```python
from build123d import *

# Parameters (mm, degrees)
SKETCH2_W           = 16
SKETCH2_H           = 14
BOSS_EXTRUDE1_DEPTH = 3
CUT_EXTRUDE1_DEPTH  = 3


with BuildPart() as part:
    # Sketch2 → Boss-Extrude1 (new body)
    with BuildSketch(Plane(origin=(0, 0, 0), x_dir=(1, 0, 0), z_dir=(0, 1, 0))):
        with Locations((-34.802547771, 15.318471338)):
            Rectangle(SKETCH2_W, SKETCH2_H)
    extrude(amount=BOSS_EXTRUDE1_DEPTH)

    # Sketch4 → Cut-Extrude1 (cut)
    with BuildSketch(Plane(origin=(0, 3, 0), x_dir=(1, 0, 0), z_dir=(0, 1, 0))):
        with BuildLine():
            Line((-41.175596086, 16.394868254), (-39.947814065, 17.622650274))
            add(Edge.make_bspline(
                [(-39.947814065, 17.622650274), (-40.733462487, 18.672629006), (-42.096388691, 18.405416924), (-42.100834752, 17.17324364), (-41.175596086, 16.394868254)],
                knots=[0, 0, 0, 0, 0.504616072, 1, 1, 1, 1], degree=3))
        make_face()
        Polygon((-39.530720652, 17.17030953), (-40.711506231, 15.989523951), (-37.03990928, 12.317927), (-34.675400844, 11.134204143), (-35.857655062, 13.500181218), align=None)
        with BuildLine():
            Line((-38.95501425, 17.722517711), (-37.627364793, 16.394868254))
            Line((-37.627364793, 16.394868254), (-37.627364793, 18.838683184))
            Line((-37.627364793, 18.838683184), (-32.457756286, 18.838683184))
            add(Edge.make_bspline(
                [(-31.400336364, 16.70034512), (-31.826000229, 16.759057378), (-32.15711446, 16.931909426), (-32.563281875, 17.99135722), (-32.457756286, 18.251227672), (-32.457756286, 18.838683184)],
                knots=[0, 0, 0, 0, 0.30144592, 0.621249631, 1, 1, 1, 1], degree=3))
            Line((-31.400336364, 16.70034512), (-30.319418222, 16.70034512))
            Line((-30.319418222, 16.70034512), (-30.319418222, 10.214836266))
            Line((-30.319418222, 10.214836266), (-37.627364793, 10.214836266))
            Line((-37.627364793, 10.214836266), (-37.627364793, 11.800966149))
            Line((-37.627364793, 11.800966149), (-38.95501425, 13.128615607))
            Line((-38.95501425, 13.128615607), (-38.95501425, 10.214836266))
            add(Edge.make_bspline(
                [(-38.95501425, 10.214836266), (-38.855731917, 8.974442118), (-37.627364793, 8.91068503)],
                knots=[0, 0, 0, 1, 1, 1], degree=2))
            Line((-37.627364793, 8.91068503), (-30.319418222, 8.91068503))
            add(Edge.make_bspline(
                [(-30.319418222, 8.91068503), (-29.146746319, 9.095747861), (-29.02114154, 10.214836266)],
                knots=[0, 0, 0, 1, 1, 1], degree=2))
            Line((-29.02114154, 10.214836266), (-29.02114154, 17.258427857))
            Line((-29.02114154, 17.258427857), (-31.929046325, 20.166332642))
            Line((-31.929046325, 20.166332642), (-37.627364793, 20.166332642))
            add(Edge.make_bspline(
                [(-37.627364793, 20.166332642), (-38.792973527, 20.218288166), (-38.95501425, 19.073665389)],
                knots=[0, 0, 0, 1, 1, 1], degree=2))
            Line((-38.95501425, 19.073665389), (-38.95501425, 17.722517711))
        make_face()
        with BuildLine():
            Line((-36.440704658, 17.558030168), (-33.773656633, 17.558030168))
            ThreePointArc((-33.773656633, 17.558030168), (-33.385935995, 17.17030953), (-33.773656633, 16.782588892))
            Line((-33.773656633, 16.782588892), (-36.440704658, 16.782588892))
            ThreePointArc((-36.440704658, 16.782588892), (-36.828425296, 17.17030953), (-36.440704658, 17.558030168))
        make_face()
        with BuildLine():
            Line((-31.517827466, 14.585505277), (-35.782754484, 14.585505277))
            Line((-35.782754484, 14.585505277), (-36.599317646, 15.402068438))
            Line((-36.599317646, 15.402068438), (-31.517827466, 15.402068438))
            add(Edge.make_bspline(
                [(-31.517827466, 14.585505277), (-30.765884411, 14.993786858), (-31.517827466, 15.402068438)],
                knots=[0, 0, 0, 1, 1, 1], degree=2))
        make_face()
        with BuildLine():
            Line((-31.517827466, 13.739569339), (-35.107180646, 13.739569339))
            Line((-35.107180646, 13.739569339), (-34.58434524, 12.881884291))
            Line((-34.58434524, 12.881884291), (-31.517827466, 12.881884291))
            add(Edge.make_bspline(
                [(-31.517827466, 12.881884291), (-30.765884411, 13.310726815), (-31.517827466, 13.739569339)],
                knots=[0, 0, 0, 1, 1, 1], degree=2))
        make_face()
        with BuildLine():
            Line((-31.517827466, 11.953704582), (-34.196624602, 11.953704582))
            Line((-34.196624602, 11.953704582), (-33.902896846, 11.134204143))
            Line((-33.902896846, 11.134204143), (-31.517827466, 11.134204143))
            add(Edge.make_bspline(
                [(-31.517827466, 11.134204143), (-30.765744911, 11.553356024), (-31.517827466, 11.953704582)],
                knots=[0, 0, 0, 1, 1, 1], degree=2))
        make_face()
    extrude(amount=-CUT_EXTRUDE1_DEPTH, mode=Mode.SUBTRACT)


solid = part.part
```
Geometry check sheet. Reference: the model listing, model coordinates, mm. Coordinates: 2 decimals unless noted, no trailing zeros. Loops run counter-clockwise (first coordinate to the right, second up) from the corner with the lowest first, then second, coordinate; pieces in that order, holes last.
Item 1: Sectioned sample at B-B, the plane x = -37.25. Record the boundary of the cut face in (y, z), then the cut area to 3 significant figures.
Item 2: Thickness scan on line 1 (Z direction, x = -33.25, y = 1); line 2 (X direction, y = 0.2, z = -10.5); line 3 (Z direction, x = -34.5, y = 0.95). Record the ranges inside material, lowest first.
Item 3: Release check for a two-part mould opening along Z. For faces 1 (the face through (-34, 2, -8.911)), 2 (the face through (-35, 1, -22.318)) record: released by +Z, released by -Z, zero draft, split by the parting line, or undercut.
Item 4: Sectioned sample at C-C, the plane y = 2. Count the separate pieces of the cut face and the enclosed holes in it, then the cut area to 3 significant figures.
Item 5: Sectioned sample at A-A, the plane z = -10.75. Record the boundary of the cut face in (x, y), then the cut area to 3 significant figures.
Check result:
1. outline: (0, -22.32) - (3, -22.32) - (3, -20.17) - (0, -20.17) - close; (0, -18.84) - (3, -18.84) - (3, -14.89) - (0, -14.89) - close; (0, -12.53) - (3, -12.53) - (3, -10.21) - (0, -10.21) - close; (0, -8.91) - (3, -8.91) - (3, -8.32) - (0, -8.32) - close
1. area: 27.0 mm2
2. line 1: z = -22.32 to -20.17, -18.84 to -15.4, -14.59 to -13.74, -12.88 to -11.95, -11.13 to -10.21, -8.91 to -8.32
2. line 2: x = -42.8 to -38.96, -37.63 to -30.32, -29.02 to -26.8
2. line 3: z = -22.32 to -20.17, -18.84 to -17.56, -16.78 to -15.4, -14.59 to -13.74, -12.88 to -10.21, -8.91 to -8.32
3. face 1: undercut
3. face 2: released by -Z
4. separate pieces: 1
4. enclosed holes: 7
4. area: 157 mm2
5. outline: (-42.8, 0) - (-38.96, 0) - (-38.96, 3) - (-42.8, 3) - close; (-37.63, 0) - (-30.32, 0) - (-30.32, 3) - (-37.63, 3) - close; (-29.02, 0) - (-26.8, 0) - (-26.8, 3) - (-29.02, 3) - close
5. area: 40.1 mm2
